Input: part model. Units: mm. Frame: model coordinates. Round coordinates to 2 decimals unless told otherwise and drop trailing zeros. Write each loop counter-clockwise with the first axis right and the second up, starting at its lowest first coordinate (ties: lowest second). Pieces come first, ordered by that corner, then holes. Notation, with made-up numbers: (-29.75, 76) -> (-22.75, 76) arc R24 cw to (-22.75, 103) -> close; hole circle Ø10 at (72.25, -20.75). An arc over 180 degrees is marked (long way). Write item = value, one per line.
Autodesk Inventor part; units mm, degrees
ref_plane "YZ Plane" through (0, 0, 0) normal (1, 0, 0) x (0, 1, 0)
ref_plane "XZ Plane" through (0, 0, 0) normal (0, 1, 0) x (-1, 0, 0)
ref_plane "XY Plane" through (0, 0, 0) normal (0, 0, 1) x (1, 0, 0)
sketch "Boceto1" plane through (0, 0, 0) normal (0, 0, 1) x (1, 0, 0)
  line L0 (0, 0) -> (400, 0)
  line L1 (400, 0) -> (400, 150)
  line L2 (400, 150) -> (0, 150)
  line L3 (0, 150) -> (0, 0)
  dimension "d0" = 150
  dimension "d1" = 400
extrude "Extrusión1" add sketch "Boceto1" along normal blind 3
sketch "Boceto3" plane through (0, 0, 3) normal (0, 0, 1) x (1, 0, 0)
  line L0 (0, 0) -> (400, 0) construction
  line L1 (400, 0) -> (400, 150) construction
  line L2 (400, 150) -> (0, 150) construction
  line L3 (0, 150) -> (0, 0) construction
  line L4 (0, 50) -> (3, 50)
  line L5 (3, 50) -> (3, 0)
  line L6 (3, 0) -> (0, 0)
  line L7 (0, 0) -> (0, 50)
  line L8 (0, 100) -> (0, 150)
  line L9 (0, 150) -> (3, 150)
  line L10 (3, 150) -> (3, 100)
  line L11 (3, 100) -> (0, 100)
  line L12 (397, 100) -> (400, 100)
  line L13 (400, 100) -> (400, 50)
  line L14 (400, 50) -> (397, 50)
  line L15 (397, 50) -> (397, 100)
  line L16 (400, 0) -> (400, 150) construction
  point P0 (400, 75)
  point P1 (400, 75)
  dimension "d15" = 3
  dimension "d16" = 50
  dimension "d19" = 100
  dimension "d24" = 3
  dimension "d25" = 50
extrude "Extrusión3" cut sketch "Boceto3" against normal blind 3
sketch "Boceto4" plane through (0, 0, 3) normal (0, 0, 1) x (1, 0, 0)
  line L0 (3, 150) -> (3, 100) construction
  line L1 (3, 100) -> (0, 100) construction
  line L2 (0, 100) -> (0, 50) construction
  line L3 (0, 50) -> (3, 50) construction
  line L4 (3, 50) -> (3, 0) construction
  line L5 (3, 0) -> (400, 0) construction
  line L6 (400, 0) -> (400, 50) construction
  line L7 (400, 50) -> (397, 50) construction
  line L8 (397, 50) -> (397, 100) construction
  line L9 (397, 100) -> (400, 100) construction
  line L10 (400, 100) -> (400, 150) construction
  line L11 (400, 150) -> (3, 150) construction
  line L12 (18, 150) -> (33, 150)
  line L13 (33, 150) -> (33, 147)
  line L14 (33, 147) -> (18, 147)
  line L15 (18, 147) -> (18, 150)
  line L16 (3, 0) -> (400, 0) construction
  line L17 (63, 147) -> (48, 147)
  line L18 (48, 147) -> (48, 150)
  line L19 (48, 150) -> (63, 150)
  line L20 (63, 150) -> (63, 147)
  line L21 (93, 147) -> (78, 147)
  line L22 (78, 147) -> (78, 150)
  line L23 (78, 150) -> (93, 150)
  line L24 (93, 150) -> (93, 147)
  line L25 (123, 147) -> (108, 147)
  line L26 (108, 147) -> (108, 150)
  line L27 (108, 150) -> (123, 150)
  line L28 (123, 150) -> (123, 147)
  line L29 (153, 147) -> (138, 147)
  line L30 (138, 147) -> (138, 150)
  line L31 (138, 150) -> (153, 150)
  line L32 (153, 150) -> (153, 147)
  line L33 (183, 147) -> (168, 147)
  line L34 (168, 147) -> (168, 150)
  line L35 (168, 150) -> (183, 150)
  line L36 (183, 150) -> (183, 147)
  line L37 (213, 147) -> (198, 147)
  line L38 (198, 147) -> (198, 150)
  line L39 (198, 150) -> (213, 150)
  line L40 (213, 150) -> (213, 147)
  line L41 (243, 147) -> (228, 147)
  line L42 (228, 147) -> (228, 150)
  line L43 (228, 150) -> (243, 150)
  line L44 (243, 150) -> (243, 147)
  line L45 (273, 147) -> (258, 147)
  line L46 (258, 147) -> (258, 150)
  line L47 (258, 150) -> (273, 150)
  line L48 (273, 150) -> (273, 147)
  line L49 (303, 147) -> (288, 147)
  line L50 (288, 147) -> (288, 150)
  line L51 (288, 150) -> (303, 150)
  line L52 (303, 150) -> (303, 147)
  line L53 (333, 147) -> (318, 147)
  line L54 (318, 147) -> (318, 150)
  line L55 (318, 150) -> (333, 150)
  line L56 (333, 150) -> (333, 147)
  line L57 (363, 147) -> (348, 147)
  line L58 (348, 147) -> (348, 150)
  line L59 (348, 150) -> (363, 150)
  line L60 (363, 150) -> (363, 147)
  line L61 (393, 147) -> (378, 147)
  line L62 (378, 147) -> (378, 150)
  line L63 (378, 150) -> (393, 150)
  line L64 (393, 150) -> (393, 147)
  line L65 (400, 150) -> (3, 150) construction
  point P0 (0, 0)
  dimension "d28" = 3
  dimension "d29" = 15
  dimension "d30" = 15
  dimension "d33" = 30
extrude "Extrusión4" cut sketch "Boceto4" against normal blind 10
properties part number "Pared1"
1) First-contact query: P1, Ø0.9, axis at y = 148.5, z = 1.5, coming from the -X side; P2, Ø1.5, axis at x = 299, z = 1.5, coming from the +Y side; P3, Ø2, axis at x = 125.5, y = 128.5, coming from the -Z side. Flat tips, straight axial feed; report the tip coordinate or a pass-through.
Solutions:
P1 = 3
P2 = 147
P3 = 0
2) Line query: L1, parallel to Y at x = 294, z = 2.4; L2, parallel to X at y = 106.5, z = 0.2; L3, parallel to X at y = 79.5, z = 0.65. Output: solid intervals per line, ascending. Write a range as from..to.
Solutions:
L1 = 0..147
L2 = 3..400
L3 = 0..397
3) Cut plane A-A (x = 176). Return the cut outline in (y, z), and give its area (3 significant figures).
Solutions:
outline = (0, 0) -> (147, 0) -> (147, 3) -> (0, 3) -> close
area = 441 mm^2
